from build123d import *

# Parameters (mm, degrees)
SKETCH_W        = 39.5
SKETCH_H        = 35
PAD_DEPTH       = 8.5
POCKET_DEPTH    = 10
POCKET001_DEPTH = 10
POCKET002_DEPTH = 8.501
CHAMFER_SIZE    = 1
CHAMFER001_SIZE = 1


with BuildPart() as part:
    # Sketch → Pad (new body)
    with BuildSketch(Plane.XZ):
        with Locations((19.75, 17.5)):
            Rectangle(SKETCH_W, SKETCH_H)
    extrude(amount=PAD_DEPTH)

    # Sketch001 (on Face2 of Pad) → Pocket (cut)
    with BuildSketch(Plane(origin=(39.5, 0, 0), x_dir=(0, 0, 1), z_dir=(1, 0, 0))):
        Polygon((4.193853, 3.239104), (3.760896, 2.806147), (3.760896, 2.193853), (4.193853, 1.760896), (4.806147, 1.760896), (5.239104, 2.193853), (5.239104, 2.806147), (4.806147, 3.239104), align=None)
        Polygon((17.193853, 3.239104), (16.760896, 2.806147), (16.760896, 2.193853), (17.193853, 1.760896), (17.806147, 1.760896), (18.239104, 2.193853), (18.239104, 2.806147), (17.806147, 3.239104), align=None)
        Polygon((30.193853, 3.239104), (29.760896, 2.806147), (29.760896, 2.193853), (30.193853, 1.760896), (30.806147, 1.760896), (31.239104, 2.193853), (31.239104, 2.806147), (30.806147, 3.239104), align=None)
    extrude(amount=-POCKET_DEPTH, mode=Mode.SUBTRACT)

    # Sketch003 (on Face2 of Pocket) → Pocket001 (cut)
    with BuildSketch(Plane(origin=(0, 0, 0), x_dir=(0, 0, -1), z_dir=(-1, 0, 0))):
        Polygon((-30.806147, 3.239104), (-31.239104, 2.806147), (-31.239104, 2.193853), (-30.806147, 1.760896), (-30.193853, 1.760896), (-29.760896, 2.193853), (-29.760896, 2.806147), (-30.193853, 3.239104), align=None)
        Polygon((-17.806147, 3.239104), (-18.239104, 2.806147), (-18.239104, 2.193853), (-17.806147, 1.760896), (-17.193853, 1.760896), (-16.760896, 2.193853), (-16.760896, 2.806147), (-17.193853, 3.239104), align=None)
        Polygon((-4.806147, 3.239104), (-5.239104, 2.806147), (-5.239104, 2.193853), (-4.806147, 1.760896), (-4.193853, 1.760896), (-3.760896, 2.193853), (-3.760896, 2.806147), (-4.193853, 3.239104), align=None)
    extrude(amount=-POCKET001_DEPTH, mode=Mode.SUBTRACT)

    # Sketch004 (on Face5 of Pocket001) → Pocket002 (cut, through all)
    with BuildSketch(Plane.XZ.offset(8.5)):
        Polygon((4.443853, 26.239104), (4.010896, 25.806147), (4.010896, 25.193853), (4.443853, 24.760896), (5.056147, 24.760896), (5.489104, 25.193853), (5.489104, 25.806147), (5.056147, 26.239104), align=None)
        Polygon((34.443853, 26.239104), (34.010896, 25.806147), (34.010896, 25.193853), (34.443853, 24.760896), (35.056147, 24.760896), (35.489104, 25.193853), (35.489104, 25.806147), (35.056147, 26.239104), align=None)
        Polygon((34.443853, 10.239104), (34.010896, 9.806147), (34.010896, 9.193853), (34.443853, 8.760896), (35.056147, 8.760896), (35.489104, 9.193853), (35.489104, 9.806147), (35.056147, 10.239104), align=None)
        Polygon((4.443853, 10.239104), (4.010896, 9.806147), (4.010896, 9.193853), (4.443853, 8.760896), (5.056147, 8.760896), (5.489104, 9.193853), (5.489104, 9.806147), (5.056147, 10.239104), align=None)
        Polygon((12.25, 4.509619), (27.25, 4.509619), (34.75, 17.5), (27.25, 30.490381), (12.25, 30.490381), (4.75, 17.5), align=None)
    extrude(amount=-POCKET002_DEPTH, mode=Mode.SUBTRACT)

    # Chamfer
    chamfer_edges = [part.edges().sort_by_distance(p)[0] for p in [
        (39.5, -4.25, 35),
        (0, -4.25, 35),
        (0, -4.25, 0),
        (39.5, -4.25, 0),
        (39.5, -8.5, 17.5),
        (19.75, -8.5, 0),
        (19.75, 0, 0),
        (39.5, 0, 17.5),
        (0, 0, 17.5),
        (0, -8.5, 17.5),
        (19.75, -8.5, 35),
        (19.75, 0, 35),
    ]]
    chamfer(chamfer_edges, length=CHAMFER_SIZE)

    # Chamfer001
    chamfer001_edges = [part.edges().sort_by_distance(p)[0] for p in [
        (31, -8.5, 11.004809),
        (19.75, -8.5, 4.509619),
        (31, -8.5, 23.995191),
        (19.75, -8.5, 30.490381),
        (8.5, -8.5, 23.995191),
        (8.5, -8.5, 11.004809),
        (8.5, 0, 23.995191),
        (19.75, 0, 30.490381),
        (31, 0, 23.995191),
        (31, 0, 11.004809),
        (19.75, 0, 4.509619),
        (8.5, 0, 11.004809),
    ]]
    chamfer(chamfer001_edges, length=CHAMFER001_SIZE)


solid = part.part
Could you check a few things on this model? Use its own coordinates, in mm. A direction names the side the tool comes from. Round coordinates to 2 decimals unless told otherwise and drop trailing zeros. Order: outer loops, then holes, each group sorted by start corner. A loop starts at its lowest first (then second) coordinate and runs counter-clockwise, first axis right, second up.
Q1. I'm going to push a flat-ended pin straight in: P1, Ø4, axis at x = 31.5, z = 20.5, coming from the -Y side. Where does the tip first touch, or does it pass through?
Geometry says:
P1: stops at y = -8.19
Q2. Which directions (+Z, -Z, +X, -X, +Y, -Y) give clear straight access to the entire face, cutting with the end or side of a thin tool? Please do faces 5 (the face through (8.552, -4.296, 24.086)), 6 (the face through (38.8, -0.6, 34.3)), 7 (the face through (19.86, -0.51, 30.98)), 8 (the face through (31.48, -7.99, 24.14)), 9 (the face through (0, -4, 17)).
Geometry says:
face 5: +Y, -Y
face 6: +Z, +X, +Y
face 7: +Y
face 8: -Y
face 9: +Z, -Z, -X, +Y, -Y
Q3. Please list where these lines run through material, in increasing order: probe 1 along Z at (x, y) = (35, -1.5); probe 2 along Z at (x, y) = (13.5, -5.5); probe 3 along Z at (x, y) = (6, -2).
Geometry says:
probe 1: z = 0 to 8.76, 10.24 to 24.76, 26.24 to 35
probe 2: z = 0 to 4.51, 30.49 to 35
probe 3: z = 0 to 3.95, 5.05 to 15.33, 19.67 to 29.95, 31.05 to 35
Q4. Thinking about a two-plate mould opening in X: for faces 1 (the face through (8.02, -7.99, 10.86)), 2 (the face through (0.7, -7.9, 34.3)), 3 (the face through (20, -4, 30.49)), 4 (the face through (39, -4.2, 0.5)), which applies, released by +X, released by -X, zero draft, split by the parting line, or undercut?
Geometry says:
face 1: undercut
face 2: released by -X
face 3: undercut
face 4: released by +X
Q5. Imagine slicing it at B-B, the plane x = 13. List the corners of the cut face in (y, z) for me.
Geometry says:
outline: (-8.5, 1) - (-7.5, 0) - (-1, 0) - (0, 1) - (0, 3.51) - (-1, 4.51) - (-7.5, 4.51) - (-8.5, 3.51) - close; (-8.5, 31.49) - (-7.5, 30.49) - (-1, 30.49) - (0, 31.49) - (0, 34) - (-1, 35) - (-7.5, 35) - (-8.5, 34) - close
Q6. Imagine slicing it at A-A, the plane z = 22. List the corners of the cut face in (x, y) for me, then the cut area to 3 significant figures.
Geometry says:
outline: (0, -7.5) - (1, -8.5) - (6.19, -8.5) - (7.35, -7.5) - (7.35, -1) - (6.19, 0) - (1, 0) - (0, -1) - close; (32.15, -7.5) - (33.31, -8.5) - (38.5, -8.5) - (39.5, -7.5) - (39.5, -1) - (38.5, 0) - (33.31, 0) - (32.15, -1) - close
area: 121 mm2
Q7. Imagine slicing it at C-C, the plane x = 8.5. State how many separate pieces and enclosed holes the cut face has, then the cut area to 3 significant figures.
Geometry says:
separate pieces: 2
enclosed holes: 2
area: 177 mm2
